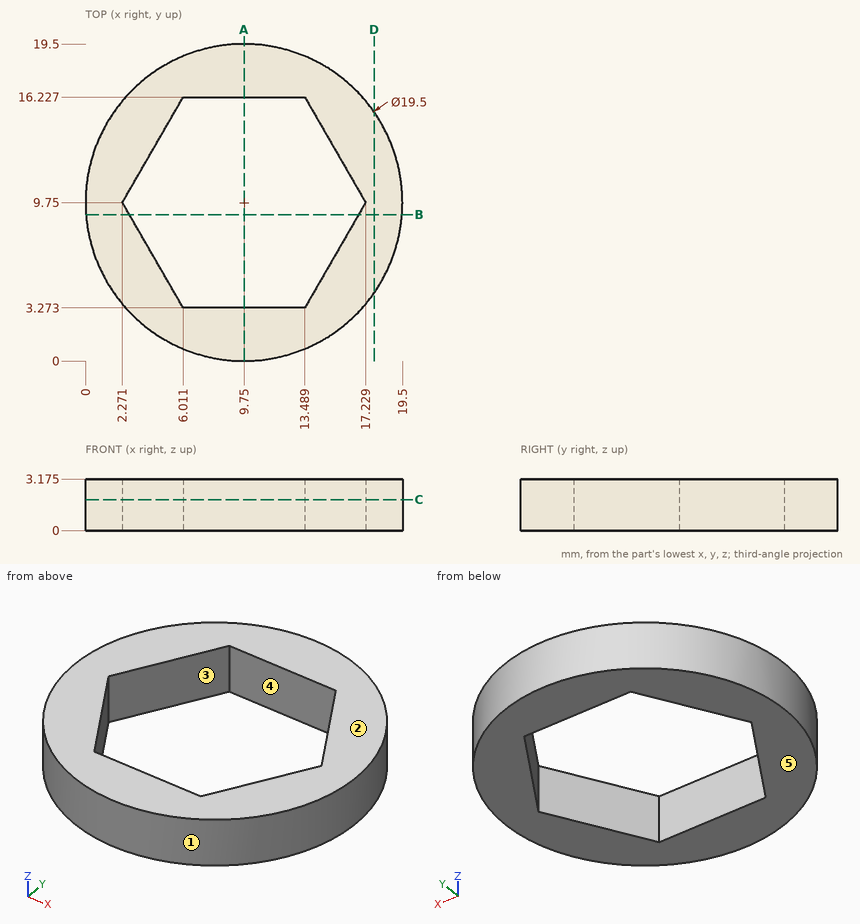
Design review of the part shown in the three views and the two pictorial views. Dimensions are in mm from the part's minimum x, y and z. A direction names the side the tool comes from. Round coordinates to 2 decimals unless told otherwise and drop trailing zeros. Write each loop counter-clockwise with the first axis right and the second up, starting at its lowest first coordinate (ties: lowest second). Pieces come first, ordered by that corner, then holes. Notation, with made-up numbers: (-32, 5) -> (1, 5) arc R23 cw to (1, 22) -> close; hole circle Ø6 at (-31, -33). An arc over 180 degrees is marked (long way). One line per question, with ' | ' between items. Start each with the question number.
1) Add section D-D (x = 17.75). Write out the cut boundary in (y, z) (1 decimal), and give its area (3 significant figures).
2) Add section B-B (y = 9). Write out the cut boundary in (x, z) (1 decimal).
3) Add section C-C (z = 1.9). Write out the cut boundary in (x, y), and give its area (3 significant figures).
4) Wall thickness on line 1 along Y through (x, z) = (9.5, 1.2); line 2 along Y through (x, z) = (10.75, 1.7); line 3 along X through (y, z) = (5, 1.8) (1 decimal): over which ranges is each line inside the solid? List them lowest first.
5) Add section A-A (x = 9.75). Write out the cut boundary in (y, z) (1 decimal).
6) For pin 1 Ø1.5 at (x, z) = (6, 3) entering from +Y; pin 2 Ø1.6 at (x, z) = (8, 2) entering from +Y, all flat-tipped, find the tip position at first contact; note any pin that passes through.
7) Machinability: for the marked faces 4 and 5, which of the approach directions +Z, -Z, +X, -X, +Y, -Y give a long, thin tool a straight path to every point of the face, cutting with its end or side? Answer none if there is none.
8) Mouldability with a two-part tool opening along X and no side actions: class the marked faces 1, 2 and 3 as +X half, -X half, draft (parallel to the pull), parting line (faces both ways), or undercut.
Reported:
1) outline: (4.2, 0) -> (15.3, 0) -> (15.3, 3.2) -> (4.2, 3.2) -> close | area: 35.4 mm²
2) outline: (0, 0) -> (2.7, 0) -> (2.7, 3.2) -> (0, 3.2) -> close; (16.8, 0) -> (19.5, 0) -> (19.5, 3.2) -> (16.8, 3.2) -> close
3) outline: circle Ø19.5 at (9.75, 9.75); hole (2.27, 9.75) -> (6.01, 3.27) -> (13.49, 3.27) -> (17.23, 9.75) -> (13.49, 16.23) -> (6.01, 16.23) -> close | area: 153 mm²
4) line 1: y = 0 to 3.27, 16.23 to 19.5 | line 2: y = 0.05 to 3.27, 16.23 to 19.45 | line 3: x = 1.2 to 5, 14.5 to 18.3
5) outline: (0, 0) -> (3.3, 0) -> (3.3, 3.2) -> (0, 3.2) -> close; (16.2, 0) -> (19.5, 0) -> (19.5, 3.2) -> (16.2, 3.2) -> close
6) pin 1: stops at y = 19.03 | pin 2: stops at y = 19.45
7) face 4: +Z, -Z | face 5: -Z, +X, -X, +Y, -Y
8) face 1: parting line | face 2: draft | face 3: undercut
